from build123d import *

# Parameters (mm, degrees)
SKETCH1_W                = 60
SKETCH1_H                = 134
BOSS_EXTRUDE1_DEPTH      = 2
M4_CLEARANCE_HOLE1_D     = 4.5
M4_CLEARANCE_HOLE1_DEPTH = 17.38
M4_CLEARANCE_HOLE1_TIP   = 1.351936393
M3_CLEARANCE_HOLE1_D     = 3.4
M3_CLEARANCE_HOLE1_DEPTH = 17.38
M3_CLEARANCE_HOLE1_TIP   = 1.021463052


with BuildPart() as part:
    # Sketch1 → Boss-Extrude1 (new body)
    with BuildSketch(Plane(origin=(0, 0, 0), x_dir=(1, 0, 0), z_dir=(0, 1, 0))):
        Rectangle(SKETCH1_W, SKETCH1_H)
    extrude(amount=BOSS_EXTRUDE1_DEPTH)

    # M4 Clearance Hole1
    with Locations(Plane(origin=(182.343359314, 2, 33.553549243), x_dir=(1, 0, 0), z_dir=(0, 1, 0))):
        with Locations((-182.343359314, 51.553549243), (-182.343359314, 15.553549243)):
            Hole(M4_CLEARANCE_HOLE1_D / 2, depth=M4_CLEARANCE_HOLE1_DEPTH)
            with Locations((0, 0, -(M4_CLEARANCE_HOLE1_DEPTH + M4_CLEARANCE_HOLE1_TIP / 2))):  # 118° drill point
                Cone(0, M4_CLEARANCE_HOLE1_D / 2, M4_CLEARANCE_HOLE1_TIP, mode=Mode.SUBTRACT)

    # M3 Clearance Hole1
    with Locations(Plane(origin=(182.343359314, 2, 33.553549243), x_dir=(1, 0, 0), z_dir=(0, 1, 0))):
        with Locations((-206.343359314, 96.553549243), (-158.343359314, 96.553549243), (-158.343359314, -29.446450757), (-206.343359314, -29.446450757)):
            Hole(M3_CLEARANCE_HOLE1_D / 2, depth=M3_CLEARANCE_HOLE1_DEPTH)
            with Locations((0, 0, -(M3_CLEARANCE_HOLE1_DEPTH + M3_CLEARANCE_HOLE1_TIP / 2))):  # 118° drill point
                Cone(0, M3_CLEARANCE_HOLE1_D / 2, M3_CLEARANCE_HOLE1_TIP, mode=Mode.SUBTRACT)


solid = part.part
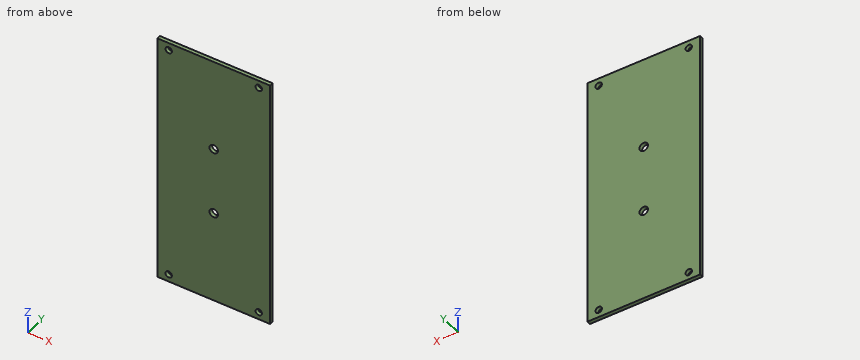
Can you work these out from the model? Positions are in its coordinate system, mm. Coordinates: 2 decimals unless noted, no trailing zeros. Order: outer loops, then holes, each group sorted by start corner. A loop starts at its lowest first (then second) coordinate and runs counter-clockwise, first axis right, second up. Notation, with made-up numbers: (8.25, 27) - (40.25, 27) arc R14 ccw to (40.25, 50) - close; hole circle Ø1 at (-34.75, 10.25). An arc over 180 degrees is marked (long way). Answer as a JSON object with one key per item and string values. Group by question number.
Q1. Imagine slicing it at B-B (z = -63). Please give me the cut outline in (x, y), and give its area (3 significant figures).
Q2. Imagine slicing it at C-C (z = 18). Please give me the cut outline in (x, y).
Q3. I need wall thicknesses on line 1 (X direction, y = 1.65, z = 63); line 2 (Z direction, x = -24, y = 1.3); line 3 (X direction, y = 0.95, z = -18). Which ranges of each line are inside material? Lowest first, please. Write a range as from..to.
Q4. Imagine slicing it at A-A (x = 24). Please give me the cut outline in (y, z), and give its area (3 significant figures).
Determined:
{
 "1": {"outline": "(-30, 0) - (-25.7, 0) - (-25.7, 2) - (-30, 2) - close; (-22.3, 0) - (22.3, 0) - (22.3, 2) - (-22.3, 2) - close; (25.7, 0) - (30, 0) - (30, 2) - (25.7, 2) - close", "area": "106 mm2"},
 "2": {"outline": "(-30, 0) - (-2.25, 0) - (-2.25, 2) - (-30, 2) - close; (2.25, 0) - (30, 0) - (30, 2) - (2.25, 2) - close"},
 "3": {"line 1": "x = -30..-25.7, -22.3..22.3, 25.7..30", "line 2": "z = -67..-64.7, -61.3..61.3, 64.7..67", "line 3": "x = -30..-2.25, 2.25..30"},
 "4": {"outline": "(0, -67) - (2, -67) - (2, -64.7) - (0, -64.7) - close; (0, -61.3) - (2, -61.3) - (2, 61.3) - (0, 61.3) - close; (0, 64.7) - (2, 64.7) - (2, 67) - (0, 67) - close", "area": "254 mm2"}
}
